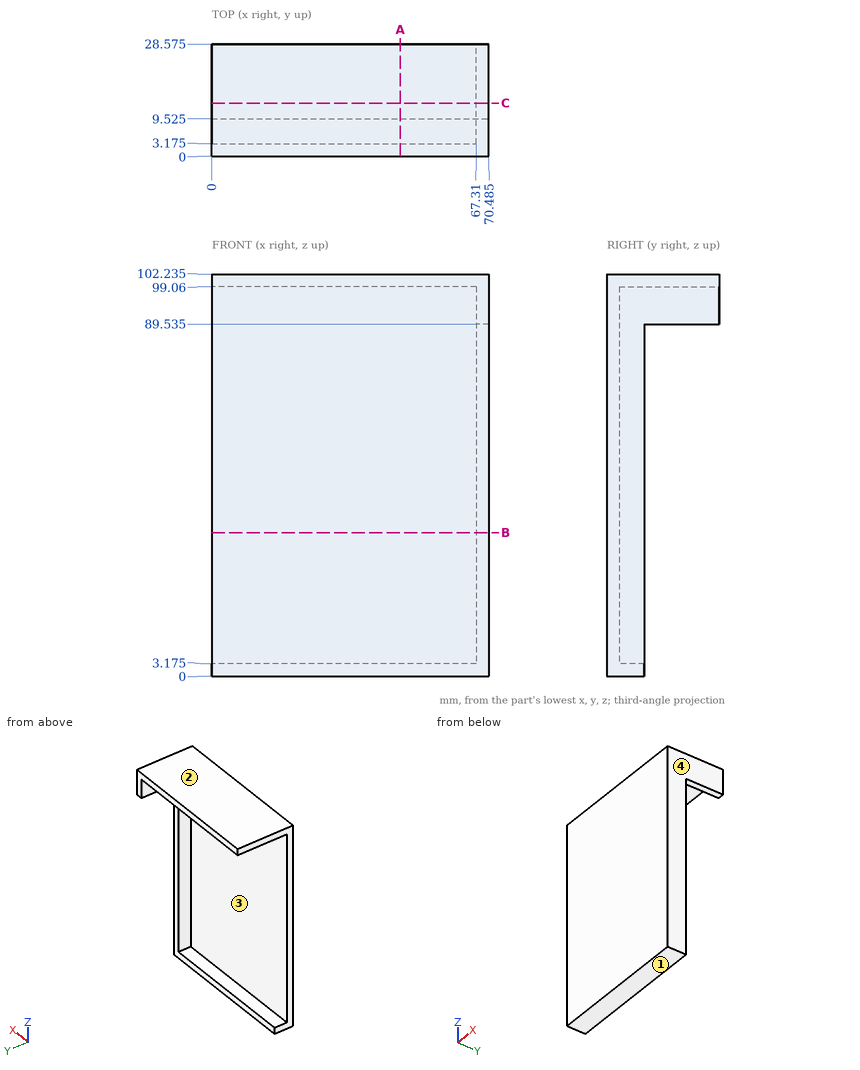
Input: dimensioned drawing with shaded views. Units: mm. Origin: part minimum x, y, z. Coordinates: 2 decimals unless noted, no trailing zeros. Write each loop counter-clockwise with the first axis right and the second up, starting at its lowest first coordinate (ties: lowest second). Pieces come first, ordered by that corner, then holes. Notation, with made-up numbers: M 51.25,-7 L 57.25,-7 A19 ccw 57.25,15 Z; hole C 12,73 d4. An arc over 180 degrees is marked long. Answer as a JSON object with one key per item and string values. Group by question number.
(1) Section B-B on z = 36.5. Output: boundary loops of the cut face in (x, y) (3 decimals).
(2) Ray query, line 1 along Z through (x, y) = (59, 8) (3 decimals); line 2 along Z through (x, y) = (4, 26.5) (3 decimals); line 3 along Y through (x, z) = (60, 51.5) (3 decimals). Return the intervals inside material, ascending. Write a range as [from, to].
(3) Section C-C on y = 13.5. Output: boundary loops of the cut face in (x, z) (3 decimals).
(4) Mould query, pull axis Z, two halves, no side actions, for the marked faces 1, 2, 3 and 4. Classes: pulls with the +Z half, pulls with the -Z half, needs draft (parallel to the pull), parting line crosses it, or undercut.
(5) Contact query for flat-ended pins moving along their axis: P1, Ø1, axis at x = 69, y = 21, coming from the -Z side (3 decimals); P2, Ø1.5, axis at y = 11.5, z = 66.5, coming from the -X side; P3, Ø1.5, axis at x = 7.5, z = 25, coming from the +Y side (3 decimals); P4, Ø6, axis at y = 6.5, z = 36, coming from the -X side. Output: stop coordinate, or through.
(6) Section A-A on x = 48. Output: boundary loops of the cut face in (y, z) (3 decimals), plus the area to 3 significant figures.
Result set:
{
 "1": {"outline": "M 0,0 L 70.485,0 L 70.485,9.525 L 67.31,9.525 L 67.31,3.175 L 0,3.175 Z"},
 "2": {"line 1": "z = [0, 3.175], [99.06, 102.235]", "line 2": "z = [99.06, 102.235]", "line 3": "y = [0, 3.175]"},
 "3": {"outline": "M 0,99.06 L 67.31,99.06 L 67.31,89.535 L 70.485,89.535 L 70.485,102.235 L 0,102.235 Z"},
 "4": {"face 1": "pulls with the -Z half", "face 2": "pulls with the +Z half", "face 3": "undercut", "face 4": "needs draft"},
 "5": {"P1": "stops at z = 89.535", "P2": "passes through", "P3": "stops at y = 3.175", "P4": "stops at x = 67.31"},
 "6": {"outline": "M 0,0 L 9.525,0 L 9.525,3.175 L 3.175,3.175 L 3.175,99.06 L 28.575,99.06 L 28.575,102.235 L 0,102.235 Z", "area": "425 mm2"}
}
